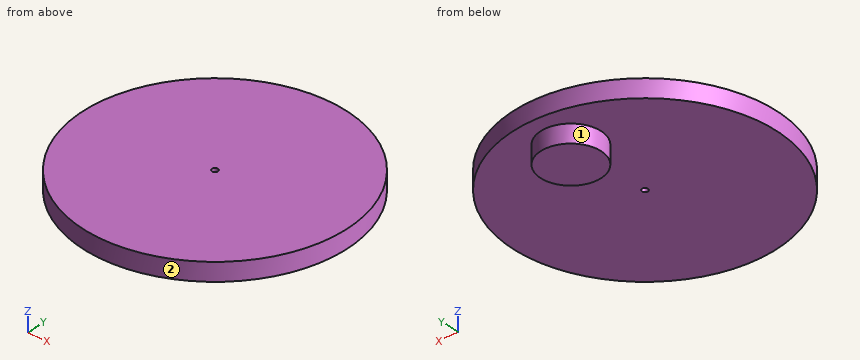
Autodesk Inventor part; units mm, degrees
ref_plane "YZ Plane" through (0, 0, 0) normal (1, 0, 0) x (0, 1, 0)
ref_plane "XZ Plane" through (0, 0, 0) normal (0, 1, 0) x (-1, 0, 0)
ref_plane "XY Plane" through (0, 0, 0) normal (0, 0, 1) x (1, 0, 0)
sketch "Sketch1" plane through (0, 0, 0) normal (0, 0, 1) x (1, 0, 0)
  circle A0 centre (0, 0) radius 21.8
  dimension "d0" = 43.6
extrude "Cuerpo" add sketch "Sketch1" along normal blind 3
sketch "Sketch2" plane through (0, 0, 0) normal (0, 0, -1) x (-1, 0, 0)
  circle A0 centre (0, 14.3) radius 5
  point P0 (0, 0)
  dimension "d4" = 14.3
  dimension "d5" = 10
extrude "Manivela" add sketch "Sketch2" along normal blind 3
sketch "Sketch3" plane through (0, 0, 0) normal (0, 0, -1) x (-1, 0, 0)
  circle A0 centre (0, 0) radius 21.8
hole "Centro" at (0, 0, 0) direction (0, 0, 1) diameter 1 end through all
equation "\"d0\" = ri_diametro"
equation "\"d1\" = ri_grosor"
equation "\"d5\" = ri_eje_diametro"
equation "\"d6\" = ri_eje_grosor"
equation "\"d8\" = ri_ancla_diametro"
properties part number "Rueda Interna"
Part model, mm, in its own coordinate system. Face numbers are marked on the shaded views. A direction names the side the tool comes from. Coordinates: 2 decimals unless noted, no trailing zeros. Write each loop counter-clockwise with the first axis right and the second up, starting at its lowest first coordinate (ties: lowest second). Pieces come first, ordered by that corner, then holes.
Item 1: Probe line 1 (Y direction, x = 0, z = 1.95); line 2 (Z direction, x = 6.5, y = 18); line 3 (Y direction, x = -9, z = 1.4). List the from-to ranges inside material, lowest first.
Item 2: Slice it at A-A (x = 0). Write the cut outline in (y, z).
Item 3: Slice it at D-D (y = 14.3). Write the cut outline in (x, z).
Item 4: Slice it at B-B (y = 0). Write the cut outline in (x, z), and give its area (3 significant figures).
Item 5: Pin check, flat tips, straight feed: pin 1 (3 mm diameter, centred on y = 9.5, z = 1.5, fed in from -X); pin 2 (12 mm diameter, centred on x = -4, y = -3, fed in from -Z); pin 3 (1 mm diameter, centred on y = -11.5, z = 2, fed in from +X); pin 4 (1.5 mm diameter, centred on x = -7.5, z = -1.5, fed in from +Y). Stop position of each tip, or through.
Item 6: Slice it at C-C (z = 1.6). Write the cut outline in (x, y), and give its area (3 significant figures).
Item 7: Which spindle directions (+Z, -Z, +X, -X, +Y, -Y) get a long thin tool onto all of the face, cutting with end or side? Do the marked faces 1 and 2. Say none if no direction does.
Results found:
1. line 1: y = -21.8 to -0.5, 0.5 to 21.8
1. line 2: z = 0 to 3
1. line 3: y = -19.86 to 19.86
2. outline: (-21.8, 0) - (-0.5, 0) - (-0.5, 3) - (-21.8, 3) - close; (0.5, 0) - (9.3, 0) - (9.3, -3) - (19.3, -3) - (19.3, 0) - (21.8, 0) - (21.8, 3) - (0.5, 3) - close
3. outline: (-16.45, 0) - (-5, 0) - (-5, -3) - (5, -3) - (5, 0) - (16.45, 0) - (16.45, 3) - (-16.45, 3) - close
4. outline: (-21.8, 0) - (-0.5, 0) - (-0.5, 3) - (-21.8, 3) - close; (0.5, 0) - (21.8, 0) - (21.8, 3) - (0.5, 3) - close
4. area: 128 mm2
5. pin 1: stops at x = -20.28
5. pin 2: stops at z = 0
5. pin 3: stops at x = 18.82
5. pin 4: passes through
6. outline: circle Ø43.6 at (0, 0); hole circle Ø1 at (0, 0)
6. area: 1,490 mm2
7. face 1: -Z
7. face 2: +Z, -Z
